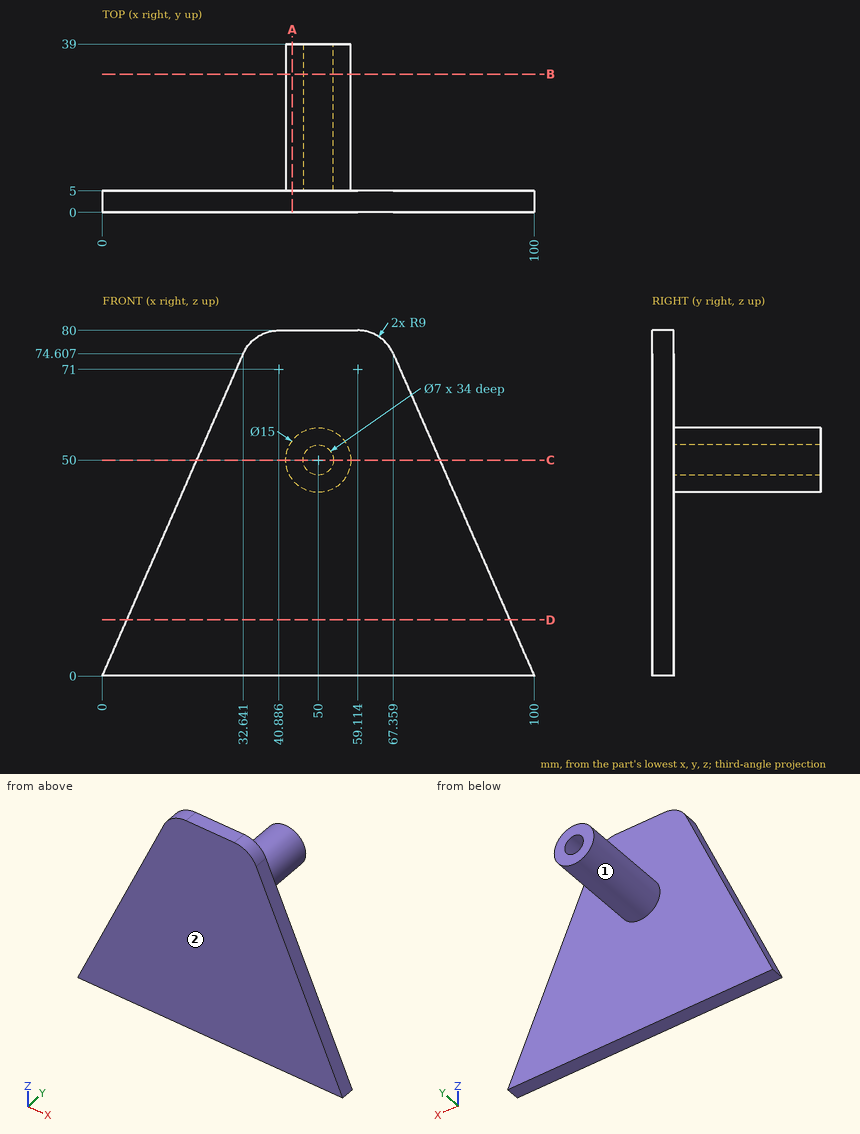
The figure shows three views and two pictorial views of one solid part (mm, origin at its lowest corner). Answer the questions. A direction names the side the tool comes from. Give positions to 0.01 mm unless a question says otherwise; leave off trailing zeros. Loops run counter-clockwise (first coordinate to the right, second up) from the corner with the lowest first, then second, coordinate; pieces in that order, holes last. Notation, with made-up numbers: (56, -31) -> (68, -31) arc R24 ccw to (68, 3) -> close; hole circle Ø11 at (28.25, 34.5). An arc over 180 degrees is marked (long way). Use a Markdown table: item, result. Add a question column.
1. Section A-A on x = 44 is taken. Determine the outline of the cut face in (y, z), and give its area (3 significant figures).
2. Section D-D on z = 13 is taken. Determine the outline of the cut face in (x, y).
3. For the marked faces 1 and 2, determine the directions among +Z, -Z, +X, -X, +Y, -Y from which every point of the face is accessible in a straight line to the end or side of a thin tool.
4. Find the intervals of material crossed by probe 1 along Z at (x, y) = (50, 21); probe 2 along Y at (x, z) = (54, 75); probe 3 along X at (y, z) = (3, 23.5), in increasing order.
5. Flat-ended cylindrical pins translate along their axes: pin 1 Ø5.5 at (x, z) = (50, 48.5) entering from +Y; pin 2 Ø12 at (x, y) = (60.5, 23) entering from +Z; pin 3 Ø10 at (y, z) = (19.5, 47.5) entering from -X; pin 4 Ø12 at (x, z) = (69, 29.5) entering from +Y. Find the tip coordinate at first contact, or state that the pin passes through.
6. Section C-C on z = 50 is taken. Determine the outline of the cut face in (x, y) (1 decimal), and give its area (3 significant figures).
7. Section B-B on y = 32 is taken. Determine the outline of the cut face in (x, z), and give its area (3 significant figures).
Results below:
| question | item | result |
|---|---|---|
| 1 | outline | (0, 0) -> (5, 0) -> (5, 45.5) -> (39, 45.5) -> (39, 54.5) -> (5, 54.5) -> (5, 80) -> (0, 80) -> close |
| 1 | area | 706 mm^2 |
| 2 | outline | (5.69, 0) -> (94.31, 0) -> (94.31, 5) -> (5.69, 5) -> close |
| 3 | face 1 | +Y |
| 3 | face 2 | +Z, -Z, +X, -X, -Y |
| 4 | probe 1 | z = 42.5 to 46.5, 53.5 to 57.5 |
| 4 | probe 2 | y = 0 to 5 |
| 4 | probe 3 | x = 10.28 to 89.72 |
| 5 | pin 1 | stops at y = 39 |
| 5 | pin 2 | stops at z = 56 |
| 5 | pin 3 | stops at x = 42.5 |
| 5 | pin 4 | stops at y = 5 |
| 6 | outline | (21.9, 0) -> (78.1, 0) -> (78.1, 5) -> (57.5, 5) -> (57.5, 39) -> (53.5, 39) -> (53.5, 5) -> (46.5, 5) -> (46.5, 39) -> (42.5, 39) -> (42.5, 5) -> (21.9, 5) -> close |
| 6 | area | 553 mm^2 |
| 7 | outline | circle Ø15 at (50, 50); hole circle Ø7 at (50, 50) |
| 7 | area | 138 mm^2 |
